Build history of the part. All positions in model axes, mm. A direction names the side the tool comes from. Round coordinates to 2 decimals unless told otherwise and drop trailing zeros. Write each loop counter-clockwise with the first axis right and the second up, starting at its lowest first coordinate (ties: lowest second). Pieces come first, ordered by that corner, then holes. Notation, with made-up numbers: M 76.5,50.5 L 128.5,50.5 A25 ccw 128.5,86.5 Z; hole C -16.5,1.5 d7. An arc over 180 degrees is marked long. Use a Markdown table: item, result.
from build123d import *

# Parameters (mm, degrees)
EXTRUDE_1_DEPTH     = 30.48
SKETCH_4_R          = 3.302
EXTRUDE_2_DEPTH     = 6.12463
SKETCH_5_W          = 82.55
SKETCH_5_H          = 48.620400001
EXTRUDE_3_DEPTH     = 3
SKETCH_6_R          = 1.5
CUT_EXTRUDE_1_DEPTH = 3
SKETCH_7_R          = 1.5
CUT_EXTRUDE_2_DEPTH = 2.5
SKETCH_8_R          = 1.5
CUT_EXTRUDE_3_DEPTH = 10
SKETCH_9_W          = 8.255
SKETCH_9_H          = 5
CUT_EXTRUDE_4_DEPTH = 19


with BuildPart() as part:
    # 스케치3 → 보스-돌출1 (new body)
    with BuildSketch(Plane.XY):
        Polygon((21517.522317655, 8422.852866974), (21525.777317655, 8422.852866974), (21525.777317655, 8382.487466973), (21591.817317655, 8382.487466973), (21591.817317655, 8422.852866974), (21600.072317655, 8422.852866974), (21600.072317655, 8374.232466973), (21517.522317655, 8374.232466973), align=None)
    extrude(amount=EXTRUDE_1_DEPTH)

    # 스케치4 → 보스-돌출2 (add)
    with BuildSketch(Plane(origin=(0, 8374.232466973, 0), x_dir=(-1, 0, 0), z_dir=(0, -1, 0))):
        with Locations((-21576.717457655, -15.24)):
            Circle(SKETCH_4_R)
    extrude(amount=EXTRUDE_2_DEPTH)

    # 스케치5 → 보스-돌출3 (add)
    with BuildSketch(Plane(origin=(0, 0, 0), x_dir=(-1, 0, 0), z_dir=(0, 0, -1))):
        with Locations((-21558.797317655, 8398.542666974)):
            Rectangle(SKETCH_5_W, SKETCH_5_H)
    extrude(amount=EXTRUDE_3_DEPTH)

    # 스케치6 → 컷-돌출1 (cut)
    with BuildSketch(Plane.XY):
        with Locations((21577.97657564, 8407.672466973)):
            Circle(SKETCH_6_R)
        with Locations((21567.97657564, 8407.672466973)):
            Circle(SKETCH_6_R)
        with Locations((21567.97657564, 8397.672466973)):
            Circle(SKETCH_6_R)
        with Locations((21577.97657564, 8397.672466973)):
            Circle(SKETCH_6_R)
    extrude(amount=-CUT_EXTRUDE_1_DEPTH, mode=Mode.SUBTRACT)

    # 스케치7 → 컷-돌출2 (cut)
    with BuildSketch(Plane.XY):
        Polygon((21569.593155483, 8410.472467064), (21566.359995798, 8410.472467064), (21564.743415955, 8407.672466973), (21566.359995798, 8404.872466883), (21569.593155483, 8404.872466883), (21571.209735325, 8407.672466973), align=None)
        with Locations((21567.97657564, 8407.672466973)):
            Circle(SKETCH_7_R, mode=Mode.SUBTRACT)
        Polygon((21569.593155483, 8400.472467064), (21566.359995798, 8400.472467064), (21564.743415955, 8397.672466973), (21566.359995798, 8394.872466883), (21569.593155483, 8394.872466883), (21571.209735325, 8397.672466973), align=None)
        with Locations((21567.97657564, 8397.672466973)):
            Circle(SKETCH_7_R, mode=Mode.SUBTRACT)
        Polygon((21579.593155483, 8400.472467064), (21576.359995798, 8400.472467064), (21574.743415955, 8397.672466973), (21576.359995798, 8394.872466883), (21579.593155483, 8394.872466883), (21581.209735325, 8397.672466973), align=None)
        with Locations((21577.97657564, 8397.672466973)):
            Circle(SKETCH_7_R, mode=Mode.SUBTRACT)
        Polygon((21579.593155483, 8410.472467064), (21576.359995798, 8410.472467064), (21574.743415955, 8407.672466973), (21576.359995798, 8404.872466883), (21579.593155483, 8404.872466883), (21581.209735325, 8407.672466973), align=None)
        with Locations((21577.97657564, 8407.672466973)):
            Circle(SKETCH_7_R, mode=Mode.SUBTRACT)
    extrude(amount=-CUT_EXTRUDE_2_DEPTH, mode=Mode.SUBTRACT)

    # 스케치8 → 컷-돌출3 (cut)
    with BuildSketch(Plane(origin=(0, 8422.852866974, 0), x_dir=(1, 0, 0), z_dir=(0, 1, 0))):
        with Locations((21597.072317655, -6)):
            Circle(SKETCH_8_R)
        with Locations((21597.072317655, -24.48)):
            Circle(SKETCH_8_R)
        with Locations((21520.522317655, -24.48)):
            Circle(SKETCH_8_R)
        with Locations((21520.522317655, -6)):
            Circle(SKETCH_8_R)
    extrude(amount=-CUT_EXTRUDE_3_DEPTH, mode=Mode.SUBTRACT)

    # 스케치9 → 컷-돌출4 (cut)
    with BuildSketch(Plane.XY.offset(30.48)):
        with Locations((21595.944817655, 8388.987466973)):
            Rectangle(SKETCH_9_W, SKETCH_9_H)
    extrude(amount=-CUT_EXTRUDE_4_DEPTH, mode=Mode.SUBTRACT)


solid = part.part
Q1. Which spindle directions (+Z, -Z, +X, -X, +Y, -Y) get a long thin tool onto all of the face, cutting with end or side? Do faces 1 (the flat face through (21565.56, 8399.09, -1.23)), 2 (the flat face through (21596, 8391.487, 21)), 3 (the flat face through (21597, 8412.853, 24)). Say none if no direction does.
Response values:
| item | result |
|---|---|
| face 1 | +Z |
| face 2 | +Z, +X |
| face 3 | +Y |
Q2. Cut at B-B on y = 8415.5. Give the cut face in (x, z).
Response values:
| item | result |
|---|---|
| outline | M 21517.52,-3 L 21600.07,-3 L 21600.07,30.48 L 21591.82,30.48 L 21591.82,0 L 21525.78,0 L 21525.78,30.48 L 21517.52,30.48 Z; hole C 21520.52,6 d3; hole C 21520.52,24.48 d3; hole C 21597.07,6 d3; hole C 21597.07,24.48 d3 |
Q3. Drop flat-ended pins along their axis: P1, Ø1.8, axis at x = 21567.98, y = 8397.67, coming from the -Z side; P2, Ø10, axis at x = 21545.5, z = 3.5, coming from the -Y side; P3, Ø3, axis at x = 21571.5, z = 14, coming from the +Y side; P4, Ø4, axis at x = 21542.5, z = 1, coming from the +Y side. Give the stop position or say it passes through.
Response values:
| item | result |
|---|---|
| P1 | passes through |
| P2 | stops at y = 8374.23 |
| P3 | stops at y = 8382.49 |
| P4 | stops at y = 8422.85 |
Q4. Cut at D-D on z = 6. Give the cut face in (x, y).
Response values:
| item | result |
|---|---|
| outline | M 21517.52,8374.23 L 21600.07,8374.23 L 21600.07,8422.85 L 21598.57,8422.85 L 21598.57,8412.85 L 21595.57,8412.85 L 21595.57,8422.85 L 21591.82,8422.85 L 21591.82,8382.49 L 21525.78,8382.49 L 21525.78,8422.85 L 21522.02,8422.85 L 21522.02,8412.85 L 21519.02,8412.85 L 21519.02,8422.85 L 21517.52,8422.85 Z |
Q5. Two-plate mould, pull along Z, no slides. Class faces 4 (the flat face through (21579, 8396, -2.5)), 5 (the cylindrical face through (21519.024, 8417.923, 5.934)), 6 (the flat face through (21578, 8400.472, -1)): +Z half, -Z half, draft (parallel to the pull), parting line (faces both ways), or undercut.
Response values:
| item | result |
|---|---|
| face 4 | +Z half |
| face 5 | undercut |
| face 6 | draft |
Q6. Cut at C-C on x = 21561.5. Give the cut face in (y, z).
Response values:
| item | result |
|---|---|
| outline | M 8374.23,-3 L 8422.85,-3 L 8422.85,0 L 8382.49,0 L 8382.49,30.48 L 8374.23,30.48 Z |
Q7. Cut at A-A on z = 20. Give the cut face in (x, y).
Response values:
| item | result |
|---|---|
| outline | M 21517.52,8374.23 L 21600.07,8374.23 L 21600.07,8386.49 L 21591.82,8386.49 L 21591.82,8382.49 L 21525.78,8382.49 L 21525.78,8422.85 L 21517.52,8422.85 Z; M 21591.82,8391.49 L 21600.07,8391.49 L 21600.07,8422.85 L 21591.82,8422.85 Z |
Q8. Drill centre lines: L1, parallel to X at y = 8421.25, z = 6; L2, parallel to X at y = 8418.5, z = 10; L3, parallel to Z at x = 21527, y = 8408. Where is each one in solid material? Low to high.
Response values:
| item | result |
|---|---|
| L1 | x = 21517.52 to 21519.02, 21522.02 to 21525.78, 21591.82 to 21595.57, 21598.57 to 21600.07 |
| L2 | x = 21517.52 to 21525.78, 21591.82 to 21600.07 |
| L3 | z = -3 to 0 |
